Design review of the part built by this model. Coordinates are the model's own, in mm. A direction names the side the tool comes from. Coordinates: 2 decimals unless noted, no trailing zeros. Answer as a JSON object with one key per item and string values.
```python
from build123d import *

# Parameters (mm, degrees)
F1_DEPTH = 381
F2_R     = 2.54
F3_R     = 2.54
F4_R     = 2.54
F5_W     = 6.35
F5_H     = 381
F6_DEPTH = 7.62
F8_DEPTH = 17.4635001


# Not quite as in the source:
# - ends of sketch curves that miss each other by under 0.0002 mm in the source are joined


with BuildPart() as f1:
    # F0 (on Top) → F1 (new body)
    with BuildSketch(Plane.XY):
        with BuildLine():
            Line((15.875, 5.55625), (15.875, 8.73125))
            Line((15.875, 8.73125), (-15.875, 8.73125))
            Line((-15.875, 8.73125), (-15.875, -0.79375))
            Line((-15.875, -0.79375), (-12.7, -0.79375))
            ThreePointArc((-12.7, -0.79375), (-9.8710707302, -6.4481459867), (-3.9751, -8.73125))
            Line((-3.9751, -8.73125), (-3.96875, -8.73125))
            ThreePointArc((-3.96875, -8.73125), (1.9312218072, -6.4502821485), (4.7625, -0.79375))
            Line((4.7625, -0.79375), (7.9375, -0.79375))
            ThreePointArc((7.9375, -0.79375), (10.9883747468, 3.5285940665), (15.875, 5.55625))
        make_face()
    extrude(amount=F1_DEPTH)

    # F2
    f2_edges = [f1.edges().sort_by_distance(p)[0] for p in [
        (7.9375, -0.79375, 190.5),
    ]]
    fillet(f2_edges, radius=F2_R)

    # F3
    f3_edges = [f1.edges().sort_by_distance(p)[0] for p in [
        (-12.7, -0.79375, 190.5),
    ]]
    fillet(f3_edges, radius=F3_R)

    # F4
    f4_edges = [f1.edges().sort_by_distance(p)[0] for p in [
        (4.7625, -0.79375, 190.5),
    ]]
    fillet(f4_edges, radius=F4_R)

    # F5 (on face) → F6 (cut)
    with BuildSketch(Plane(origin=(0, 8.73125, 0), x_dir=(-1, 0, 0), z_dir=(0, 1, 0))):
        with Locations((12.7, 190.5)):
            Rectangle(F5_W, F5_H)
    extrude(amount=-F6_DEPTH, mode=Mode.SUBTRACT)

    # F7 (on face) → F8 (cut, through all)
    with BuildSketch(Plane(origin=(0, 8.73125, 0), x_dir=(-1, 0, 0), z_dir=(0, 1, 0))):
        Polygon((15.875, 0), (15.875, 31.75), (-15.875, 0), align=None)
        Polygon((15.875, 381), (-15.875, 381), (15.875, 349.25), align=None)
    extrude(amount=-F8_DEPTH, mode=Mode.SUBTRACT)


solid = f1.part
```
(1) To check wall thickness, follow line 1 (Y direction, x = -4.5, z = 291); line 2 (Y direction, x = 8.5, z = 112); line 3 (X direction, y = 1.75, z = 209) (3 decimals). State the ranges of each line that lie inside material, in increasing order. Write a range as from..to.
Solved:
{"line 1": "y = -8.72..8.73", "line 2": "y = 0.51..8.73", "line 3": "x = -9.525..9.277"}
(2) For pin 1 (2 mm diameter, centred on x = -1.5, y = 2.5, fed in from +Z) (3 decimals); pin 2 (5 mm diameter, centred on y = 1, z = 342, fed in from +X); pin 3 (6 mm diameter, centred on x = 3.5, y = -0.5, fed in from +Z) (3 decimals), all flat-tipped, find the tip position at first contact; note any pin that passes through.
Solved:
{"pin 1": "stops at z = 364.625", "pin 2": "stops at x = 10.95", "pin 3": "stops at z = 371.625"}
(3) Tool access review of faces 1 (the face through (-13, 1.111, 193)), 2 (the face through (3, 8.731, 188)): name each direction out of +Z, -Z, +X, -X, +Y, -Y from which nothing blocks a thin tool from reaching the whole face with its end or side.
Solved:
{"face 1": "+Z, -Z, -X, +Y", "face 2": "+Z, -Z, +X, -X, +Y"}
